```python
from build123d import *

# Parameters (mm, degrees)
SKETCH2_R          = 2.5
CUT_EXTRUDE1_DEPTH = 4
SKETCH3_R          = 3.3
CUT_EXTRUDE2_DEPTH = 10.5
CHAMFER1_SIZE      = 1


with BuildPart() as part:
    # Sketch1 → Revolve1 (revolve)
    with BuildSketch(Plane.XY, mode=Mode.PRIVATE) as revolve1_sk:
        Polygon((0, 30), (6, 30), (6, 24), (7, 24), (7, 20), (18, 20), (18, 6), (6, 6), (6, 7.5), (0, 7.5), align=None)
    revolve(revolve1_sk.sketch.rotate(Axis((0, 0, 0), (1, 0, 0)), 90), axis=Axis((0, 0, 0), (1, 0, 0)))

    # Sketch2 → Cut-Extrude1 (cut)
    with BuildSketch(Plane.ZY):
        with Locations((0, 20)):
            Circle(SKETCH2_R)
        with Locations((17.320508076, 10)):
            Circle(SKETCH2_R)
        with Locations((17.320508076, -10)):
            Circle(SKETCH2_R)
        with Locations((0, -20)):
            Circle(SKETCH2_R)
        with Locations((-17.320508076, -10)):
            Circle(SKETCH2_R)
        with Locations((-17.320508076, 10)):
            Circle(SKETCH2_R)
    extrude(amount=-CUT_EXTRUDE1_DEPTH, mode=Mode.SUBTRACT)

    # Sketch3 → Cut-Extrude2 (cut)
    with BuildSketch(Plane(origin=(18, 0, 0), x_dir=(0, 0, -1), z_dir=(1, 0, 0))):
        with Locations((0, 12)):
            Circle(SKETCH3_R)
        with Locations((11.412678196, 3.708203932)):
            Circle(SKETCH3_R)
        with Locations((7.053423028, -9.708203932)):
            Circle(SKETCH3_R)
        with Locations((-7.053423028, -9.708203932)):
            Circle(SKETCH3_R)
        with Locations((-11.412678196, 3.708203932)):
            Circle(SKETCH3_R)
    extrude(amount=-CUT_EXTRUDE2_DEPTH, mode=Mode.SUBTRACT)

    # Chamfer1
    chamfer1_edges = [part.edges().sort_by_distance(p)[0] for p in [
        (18, 12, 3.3),
        (18, 3.708203932, -8.112678196),
        (18, -9.708203932, -3.753423028),
        (18, -9.708203932, 10.353423028),
        (18, 3.708203932, 14.712678196),
    ]]
    chamfer(chamfer1_edges, length=CHAMFER1_SIZE)


solid = part.part
```
Design review of the part built by this model. Coordinates are the model's own, in mm. A direction names the side the tool comes from. Coordinates: 2 decimals unless noted, no trailing zeros. Loops run counter-clockwise (first coordinate to the right, second up) from the corner with the lowest first, then second, coordinate; pieces in that order, holes last. Notation, with made-up numbers: (7.25, -20) - (44.25, -20) arc R11 ccw to (44.25, -10) - close; hole circle Ø4 at (50, 13). An arc over 180 degrees is marked (long way). Use CSV: the item, a comma, the result in double quotes. Start each with the question number.
1) Consider section B-B on x = 14.75. Write out the cut boundary in (y, z), then the cut area to 3 significant figures.
2) Tool access review of faces 4 (the cylindrical face through (11.916, -1.802, 5.723)), 5 (the cylindrical face through (1.97, 22.48, -0.33)), 6 (the cylindrical face through (12.32, 8.78, 0.72)): name each direction out of +Z, -Z, +X, -X, +Y, -Y from which nothing blocks a thin tool from reaching the whole face with its end or side.
3) Consider section D-D on x = 5. Write out the cut boundary in (y, z).
4) Consider section C-C on y = -4. Write out the cut boundary in (x, z), then the cut area to 3 significant figures.
5) The part is to be moulded in two halves that separate along Z. For faces 1 (the cylindrical face through (12.317, -6.436, -6.624)), 2 (the flat face through (6, -20.1, -13.5)), 3 (the cylindrical face through (1.97, -17.89, 1.34)), say which applies: +Z half, -Z half, draft (parallel to the pull), parting line (faces both ways), or undercut.
6) For pin 1 Ø1 at (y, z) = (11.5, 20.5) entering from +X; pin 2 Ø1 at (x, z) = (2.5, -4.5) entering from -Y; pin 3 Ø5 at (y, z) = (4.5, 13.5) entering from -X; pin 4 Ø1 at (x, y) = (2, 8) entering from +Z, all flat-tipped, find the tip position at first contact; note any pin that passes through.
7) Wall thickness on L1, parallel to Y at x = 12.75, z = 0; L2, parallel to Y at x = 1.6, z = 0; L3, parallel to Z at x = 2.75, y = 9: over which ranges is each line inside the solid? List them lowest first. Write a range as from..to.
Geometry says:
1,outline,"circle Ø40 at (0, 0); hole circle Ø6.6 at (-9.71, -7.05); hole circle Ø6.6 at (-9.71, 7.05); hole circle Ø12 at (0, 0); hole circle Ø6.6 at (3.71, -11.41); hole circle Ø6.6 at (3.71, 11.41); hole circle Ø6.6 at (12, 0)"
1,area,"972 mm^2"
2,face 4,"+X, -X"
2,face 5,"-X"
2,face 6,"+X"
3,outline,"circle Ø60 at (0, 0); hole circle Ø15 at (0, 0)"
4,outline,"(0, -29.73) - (6, -29.73) - (6, -23.66) - (7, -23.66) - (7, -19.6) - (18, -19.6) - (18, -4.47) - (6, -4.47) - (6, -6.34) - (0, -6.34) - close; (0, 6.34) - (6, 6.34) - (6, 4.47) - (18, 4.47) - (18, 19.6) - (7, 19.6) - (7, 23.66) - (6, 23.66) - (6, 29.73) - (0, 29.73) - close"
4,area,"652 mm^2"
5,face 1,"undercut"
5,face 2,"draft"
5,face 3,"undercut"
6,pin 1,"x = 7"
6,pin 2,"y = -29.73"
6,pin 3,"x = 0"
6,pin 4,"z = 29.05"
7,L1,"-20..-6, 6..8.7, 15.3..20"
7,L2,"-30..-22.5, -17.5..-7.5, 7.5..17.5, 22.5..30"
7,L3,"-28.62..-19.61, -15.03..15.03, 19.61..28.62"
